from build123d import *

# Parameters (mm, degrees)
SKETCH_1_R          = 24
EXTRUDE_1_DEPTH     = 5
SKETCH_2_W          = 10
SKETCH_2_H          = 15
EXTRUDE_2_DEPTH     = 15
CUT_EXTRUDE_1_REACH = 42.522
SKETCH_3_R          = 1.75
SKETCH_4_W          = 20
SKETCH_4_H          = 10
CUT_EXTRUDE_2_DEPTH = 5
F_3_0MM_1_D         = 3
FILLET_1_R          = 4


with BuildPart() as part:
    # 草图1 → 凸台-拉伸1 (new body)
    with BuildSketch(Plane(origin=(0, 0, 0), x_dir=(1, 0, 0), z_dir=(0, 1, 0))):
        with Locations(Location((0, 0, 0), (0, 0, 270))):
            Circle(SKETCH_1_R)
    extrude(amount=EXTRUDE_1_DEPTH)

    # 草图2 → 凸台-拉伸2 (add)
    with BuildSketch(Plane(origin=(0, 0, 0), x_dir=(1, 0, 0), z_dir=(0, 1, 0))):
        Rectangle(SKETCH_2_W, SKETCH_2_H)
    extrude(amount=EXTRUDE_2_DEPTH)

    # 草图3 → 切除-拉伸1 (cut, up to next)
    with BuildSketch(Plane.ZY.offset(5), mode=Mode.PRIVATE) as cut_extrude_1_sk1:
        with Locations((0, 10)):
            Circle(SKETCH_3_R)
    cut_extrude_1_tool1 = extrude(cut_extrude_1_sk1.sketch, amount=-CUT_EXTRUDE_1_REACH, mode=Mode.PRIVATE) & part.part
    add(cut_extrude_1_tool1.solids().sort_by_distance((-5, 10, 0))[0], mode=Mode.SUBTRACT)

    # 草图4 → 切除-拉伸2 (cut)
    with BuildSketch(Plane.ZY.offset(5)):
        with Locations((0, 10)):
            Rectangle(SKETCH_4_W, SKETCH_4_H)
    extrude(amount=-CUT_EXTRUDE_2_DEPTH, mode=Mode.SUBTRACT)

    # Ø3.0mm 暗销孔1 (through all)
    with Locations(Plane.XZ):
        with Locations((14, 14), (14, -14), (-14, 14), (-14, -14)):
            Hole(F_3_0MM_1_D / 2)

    # 圆角1
    fillet_1_edges = [part.edges().sort_by_distance(p)[0] for p in [
        (2.5, 15, -7.5),
        (2.5, 15, 7.5),
    ]]
    fillet(fillet_1_edges, radius=FILLET_1_R)


solid = part.part
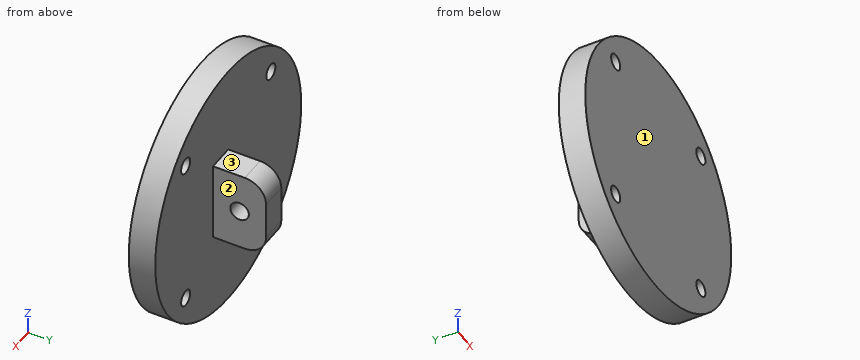
Geometry check sheet. Reference: the model listing, model coordinates, mm. Face numbers are marked on the shaded views. A direction names the side the tool comes from. Give positions to 0.01 mm unless a question says otherwise; leave off trailing zeros. Order: outer loops, then holes, each group sorted by start corner. A loop starts at its lowest first (then second) coordinate and runs counter-clockwise, first axis right, second up. Notation, with made-up numbers: (45, -36.5) - (102, -36.5) arc R20 cw to (102, 2.5) - close; hole circle Ø3 at (-23.5, 89.5). An arc over 180 degrees is marked (long way). Use one line per item in the form item = value.
1) Access from +Z, -Z, +X, -X, +Y, -Y to the whole of each face (thin tool, end or side, straight path). Record for the marked faces 1, 2 and 3.
Working result:
face_1 = +Z, -Z, +X, -X, -Y
face_2 = +Z, -Z, +X, +Y
face_3 = +Z, +X, -X, +Y
2) Depth check by flat-ended pin: pin 1 Ø3 at (y, z) = (9.5, -7) entering from -X; pin 2 Ø5.5 at (x, y) = (2.5, 7.5) entering from -Z; pin 3 Ø3.5 at (x, z) = (14, 14) entering from +Y. Enter the tip coordinate at first touch or a pass-through.
Working result:
pin_1 = 0
pin_2 = -23.96
pin_3 = 5
3) Sectioned sample at B-B (z = 0). Record the boundary of the cut face in (x, y).
Working result:
outline = (-24, 0) - (24, 0) - (24, 5) - (5, 5) - (5, 8.25) - (0, 8.25) - (0, 5) - (-24, 5) - close; (0, 11.75) - (5, 11.75) - (5, 15) - (0, 15) - close
4) Material ranges on probe 1 along Z at (x, y) = (-14, 1.8); probe 2 along Y at (x, z) = (1, 0); probe 3 along Y at (x, z) = (-13.5, 1.5), recorded low to high. Write a range as from..to.
Working result:
probe_1 = -19.49..-15.5, -12.5..12.5, 15.5..19.49
probe_2 = 0..8.25, 11.75..15
probe_3 = 0..5
5) Sectioned sample at C-C (z = 14). Record the boundary of the cut face in (x, y).
Working result:
outline = (-19.49, 0) - (-15.5, 0) - (-15.5, 5) - (-19.49, 5) - close; (-12.5, 0) - (12.5, 0) - (12.5, 5) - (-12.5, 5) - close; (15.5, 0) - (19.49, 0) - (19.49, 5) - (15.5, 5) - close
6) Sectioned sample at A-A (y = 10). Record the boundary of the cut face in (x, z), and give its area (3 significant figures).
Working result:
outline = (0, -7.5) - (5, -7.5) - (5, -1.75) - (0, -1.75) - close; (0, 1.75) - (5, 1.75) - (5, 7.5) - (0, 7.5) - close
area = 57.5 mm^2
7) Sectioned sample at D-D (x = 2). Record the boundary of the cut face in (y, z).
Working result:
outline = (0, -23.92) - (5, -23.92) - (5, -7.5) - (11, -7.5) arc R4 ccw to (15, -3.5) - (15, 3.5) arc R4 ccw to (11, 7.5) - (5, 7.5) - (5, 23.92) - (0, 23.92) - close; hole circle Ø3.5 at (10, 0)
